from build123d import *

# Parameters (mm, degrees)
SKETCH_1_R          = 9
SKETCH_1_R_2        = 6
EXTRUDE_1_DEPTH     = 2
SKETCH_2_R          = 8.7
SKETCH_2_R_2        = 6.3
CUT_EXTRUDE_1_DEPTH = 0.3


with BuildPart() as part:
    # 草图1 → 凸台-拉伸1 (new, symmetric)
    with BuildSketch(Plane.XY):
        Circle(SKETCH_1_R)
        Circle(SKETCH_1_R_2, mode=Mode.SUBTRACT)
    extrude(amount=EXTRUDE_1_DEPTH, both=True)

    # 草图2 → 切除-拉伸1 (cut)
    with BuildSketch(Plane.XY.offset(2)):
        Circle(SKETCH_2_R)
        Circle(SKETCH_2_R_2, mode=Mode.SUBTRACT)
    cut_extrude_1 = extrude(amount=-CUT_EXTRUDE_1_DEPTH, mode=Mode.SUBTRACT)

    # 镜向1: 切除-拉伸1 across plane
    add(cut_extrude_1.mirror(Plane.XY), mode=Mode.SUBTRACT)


solid = part.part
Check sheet for the modelled part. Datum: model origin and axes. Units: mm. A direction names the side the tool comes from. Coordinates: 2 decimals unless noted, no trailing zeros. Write each loop counter-clockwise with the first axis right and the second up, starting at its lowest first coordinate (ties: lowest second). Pieces come first, ordered by that corner, then holes. Notation, with made-up numbers: M 4,38.5 L 34,38.5 A10 cw 34,46.5 Z; hole C -38.5,66 d1. An arc over 180 degrees is marked long. Answer as CSV lines item,"result".
Q1. Cross-section at C-C (z = -0.2). Record the boundary of the cut face in (x, y).
Check result:
outline,"C 0,0 d18; hole C 0,0 d12"
Q2. Go/stop test with flat-tipped pins: pin 1 (1 mm diameter, centred on x = 4.5, z = -1.5, fed in from -Y); pin 2 (1.5 mm diameter, centred on x = 1.5, y = 3.5, fed in from -Z); pin 3 (1.5 mm diameter, centred on y = -5, z = 0.5, fed in from +X). Record where each tip stops, or that it passes through.
Check result:
pin 1,"y = -8.06"
pin 2,"through"
pin 3,"x = 7.93"
Q3. Mould release check, pull along X, two halves, no side actions. Record for faces 4 (the face through (-1.172, 8.923, 0.028)), 5 (the face through (-1.37, -6.15, -1.85)): released by +X, released by -X, zero draft, split by the parting line, or undercut.
Check result:
face 4,"split by the parting line"
face 5,"undercut"
Q4. Material ranges on probe 1 along Y at (x, z) = (0, 1.95); probe 2 along Y at (x, z) = (0, 0.85); probe 3 along X at (y, z) = (-0.75, 1.75), recorded low to high. Write a range as from..to.
Check result:
probe 1,"-9..-8.7, -6.3..-6, 6..6.3, 8.7..9"
probe 2,"-9..-6, 6..9"
probe 3,"-8.97..-8.67, -6.26..-5.95, 5.95..6.26, 8.67..8.97"
Q5. Cross-section at A-A (x = 0). Record the boundary of the cut face in (y, z), then the cut area to 3 significant figures.
Check result:
outline,"M -9,-2 L -8.7,-2 L -8.7,-1.7 L -6.3,-1.7 L -6.3,-2 L -6,-2 L -6,2 L -6.3,2 L -6.3,1.7 L -8.7,1.7 L -8.7,2 L -9,2 Z; M 6,-2 L 6.3,-2 L 6.3,-1.7 L 8.7,-1.7 L 8.7,-2 L 9,-2 L 9,2 L 8.7,2 L 8.7,1.7 L 6.3,1.7 L 6.3,2 L 6,2 Z"
area,"21.1 mm^2"
Q6. Set-up check for faces 1 (the face through (6, 3, -1.7)), 2 (the face through (-6, 0, 0)), 3 (the face through (-1.37, -6.15, 1.85)): record each of +Z, -Z, +X, -X, +Y, -Y from which the full face is reachable in a straight line by a thin tool's end or side.
Check result:
face 1,"-Z"
face 2,"+Z, -Z"
face 3,"+Z"
Q7. Cross-section at D-D (x = 7.25). Record the boundary of the cut face in (y, z), then the cut area to 3 significant figures.
Check result:
outline,"M -5.33,-2 L -4.81,-2 L -4.81,-1.7 L 4.81,-1.7 L 4.81,-2 L 5.33,-2 L 5.33,2 L 4.81,2 L 4.81,1.7 L -4.81,1.7 L -4.81,2 L -5.33,2 Z"
area,"36.9 mm^2"
